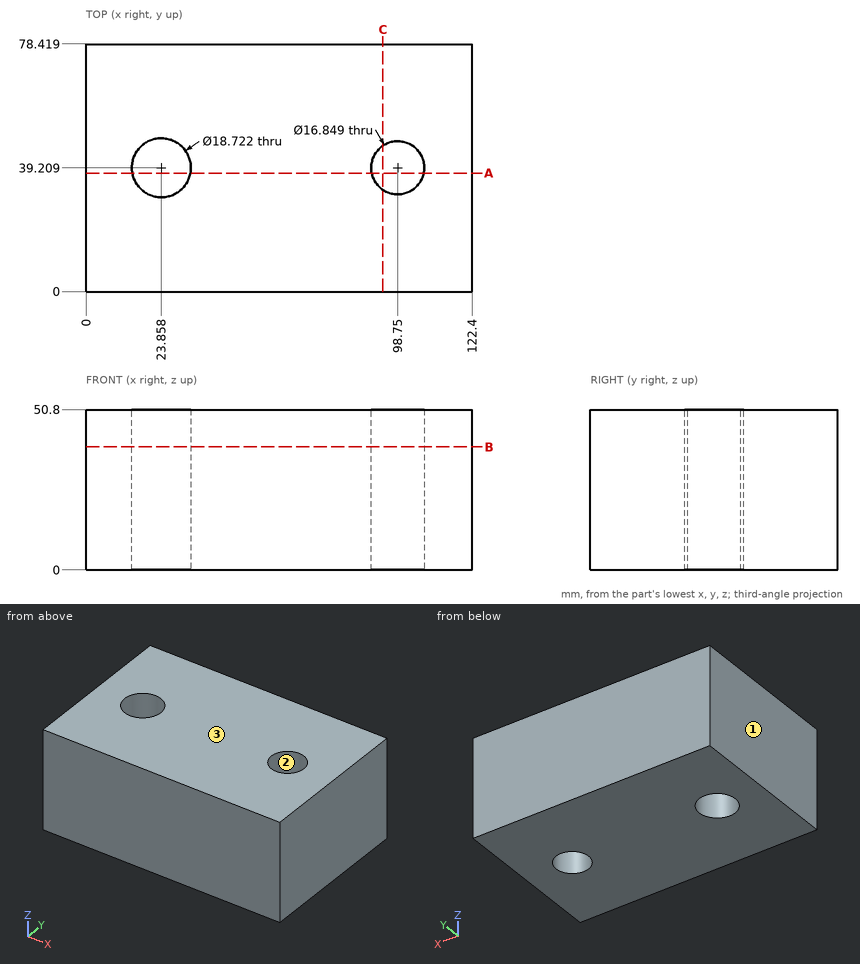
For this review, use the dimensioned drawing (mm, ordinates from the lowest corner) and the shaded views. Coordinates: 2 decimals unless noted, no trailing zeros. Order: outer loops, then holes, each group sorted by start corner. A loop starts at its lowest first (then second) coordinate and runs counter-clockwise, first axis right, second up. Notation, with made-up numbers: (49, -26) -> (94, -26) arc R35 ccw to (94, 13) -> close; hole circle Ø3 at (9.5, 56). An arc over 180 degrees is marked (long way). One line per item, written item: value. Start each with the question number.
Q1. For probe 1 along X at (y, z) = (34, 46) (1 decimal); probe 2 along X at (y, z) = (32, 8.5) (1 decimal), list the stretches that pass through material, from the lowest coordinate up.
Q2. Take a section at C-C, the plane x = 94. State the section outline as (y, z) points.
Q3. Take a section at A-A, the plane y = 37.5. State the section outline as (x, z) points (1 decimal).
Q4. Mouldability with a two-part tool opening along X and no side actions: class the marked faces 1, 2 and 3 as pulls with the +X half, pulls with the -X half, needs draft (parallel to the pull), parting line crosses it, or undercut.
Q5. Take a section at B-B, the plane z = 39. Give the number of separate pieces and of enclosed holes in the cut face, then the cut area to 3 significant figures.
Values follow:
1. probe 1: x = 0 to 16.1, 31.6 to 92.1, 105.4 to 122.4
1. probe 2: x = 0 to 17.9, 29.8 to 94.4, 103.1 to 122.4
2. outline: (0, 0) -> (32.25, 0) -> (32.25, 50.8) -> (0, 50.8) -> close; (46.17, 0) -> (78.42, 0) -> (78.42, 50.8) -> (46.17, 50.8) -> close
3. outline: (0, 0) -> (14.7, 0) -> (14.7, 50.8) -> (0, 50.8) -> close; (33.1, 0) -> (90.5, 0) -> (90.5, 50.8) -> (33.1, 50.8) -> close; (107, 0) -> (122.4, 0) -> (122.4, 50.8) -> (107, 50.8) -> close
4. face 1: pulls with the -X half
4. face 2: undercut
4. face 3: needs draft
5. separate pieces: 1
5. enclosed holes: 2
5. area: 9,100 mm2
